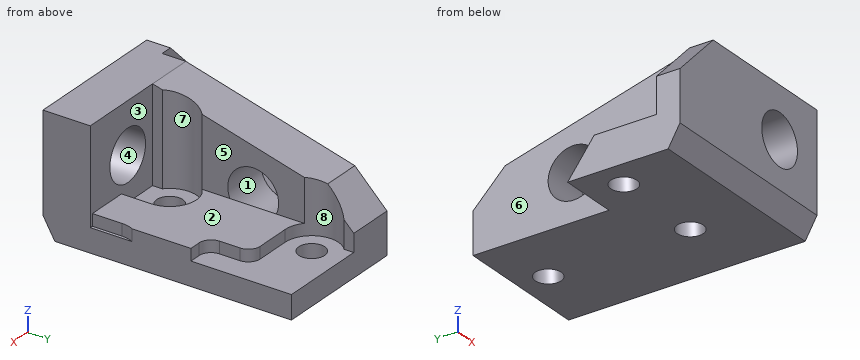
```python
from build123d import *

# Parameters (mm, degrees)
SKETCH_1_W               = 23
SKETCH_1_H               = 17
SKETCH_1_R               = 1.1
EXTRUDE_1_DEPTH          = 3
EXTRUDE_2_DEPTH          = 6
CUT_EXTRUDE_1_DEPTH      = 23.349496639
CUT_EXTRUDE_1_DEPTH_BACK = 1
SKETCH_3_R               = 2.25
CUT_EXTRUDE_2_REACH      = 24.349
SKETCH_4_W               = 4.5
SKETCH_4_H               = 17
CUT_EXTRUDE_3_DEPTH      = 2
SKETCH_6_R               = 2.15
CUT_EXTRUDE_4_DEPTH      = 4
SKETCH_7_W               = 16.5
SKETCH_7_H               = 10
EXTRUDE_3_DEPTH          = 4
SKETCH_8_R               = 2.15
CUT_EXTRUDE_5_DEPTH      = 4
CHAMFER_1_SIZE           = 1
CHAMFER_1_SIZE2          = 1.732050808
CHAMFER_2_SIZE           = 4
CUT_EXTRUDE_6_DEPTH      = 1
FILLET_1_R               = 2
CUT_EXTRUDE_7_REACH      = 21.881
FILLET_2_R               = 1
CHAMFER_3_SIZE           = 2
CHAMFER_3_SIZE2          = 2.813680863
CUT_EXTRUDE_8_REACH      = 27.729
SKETCH_11_W              = 5
SKETCH_11_H              = 10
EXTRUDE_4_DEPTH          = 5
CUT_EXTRUDE_9_REACH      = 21.222
SKETCH_13_R              = 1.1
SKETCH_14_R              = 2.25
CUT_EXTRUDE_10_DEPTH     = 1
EXTRUDE_6_REACH          = 26.135
FILLET_3_R               = 2
SKETCH_15_W              = 5
SKETCH_15_H              = 2
EXTRUDE_5_DEPTH          = 7
CUT_EXTRUDE_11_DEPTH     = 5
CHAMFER_4_SIZE           = 4


with BuildPart() as part:
    # 草图1 → 凸台-拉伸1 (new body)
    with BuildSketch(Plane.XY):
        with Locations((4, 6)):
            Rectangle(SKETCH_1_W, SKETCH_1_H)
        Circle(SKETCH_1_R, mode=Mode.SUBTRACT)
        with Locations((8, 0)):
            Circle(SKETCH_1_R, mode=Mode.SUBTRACT)
        with Locations((0, 12)):
            Circle(SKETCH_1_R, mode=Mode.SUBTRACT)
        with Locations((8, 12)):
            Circle(SKETCH_1_R, mode=Mode.SUBTRACT)
    extrude(amount=EXTRUDE_1_DEPTH)

    # 草图2 → 凸台-拉伸2 (add)
    with BuildSketch(Plane.ZY.offset(7.5)):
        Polygon((5.5, 14.5), (10, -2.5), (5.5, -2.5), (0, -2.5), (0, 14.5), align=None)
    extrude(amount=-EXTRUDE_2_DEPTH)

    # 草图3 → 切除-拉伸1 (cut, two sides: drawn at the far end of the back side and taken through both)
    with BuildSketch(Plane.XY.offset(3).offset(-CUT_EXTRUDE_1_DEPTH_BACK)):
        with Locations(Location((0, 12, 0), (0, 0, 228.189685104))):
            Circle(SKETCH_3_R)
        with Locations((8, 12)):
            Circle(SKETCH_3_R)
        with Locations(Location((0, 0, 0), (0, 0, 131.810314896))):
            Circle(SKETCH_3_R)
        with Locations((8, 0)):
            Circle(SKETCH_3_R)
    extrude(amount=CUT_EXTRUDE_1_DEPTH + CUT_EXTRUDE_1_DEPTH_BACK, mode=Mode.SUBTRACT)

    # 草图4 → 切除-拉伸2 (cut, up to next)
    with BuildSketch(Plane.XY.offset(3), mode=Mode.PRIVATE) as cut_extrude_2_sk1:
        with Locations((13.25, 6)):
            Rectangle(SKETCH_4_W, SKETCH_4_H)
    cut_extrude_2_tool1 = extrude(cut_extrude_2_sk1.sketch, amount=-CUT_EXTRUDE_2_REACH, mode=Mode.PRIVATE) & part.part
    add(cut_extrude_2_tool1.solids().sort_by_distance((13.25, 6, 3))[0], mode=Mode.SUBTRACT)

    # 草图5 → 切除-拉伸3 (cut)
    with BuildSketch(Plane.ZY.offset(7.5)):
        Polygon((0, 14.5), (0, -2.5), (10, -2.5), (5.5, 14.5), align=None)
    extrude(amount=-CUT_EXTRUDE_3_DEPTH, mode=Mode.SUBTRACT)

    # 草图6 → 切除-拉伸4 (cut)
    with BuildSketch(Plane.ZY.offset(5.5)):
        with Locations(Location((3.875, 6, 0), (0, 0, 270))):
            Circle(SKETCH_6_R)
    extrude(amount=-CUT_EXTRUDE_4_DEPTH, mode=Mode.SUBTRACT)

    # 草图7 → 凸台-拉伸3 (add)
    with BuildSketch(Plane.XZ.offset(2.5)):
        with Locations((2.75, 5)):
            Rectangle(SKETCH_7_W, SKETCH_7_H)
    extrude(amount=EXTRUDE_3_DEPTH)

    # 草图8 → 切除-拉伸5 (cut)
    with BuildSketch(Plane.XZ.offset(6.5)):
        with Locations(Location((1.5, 5.7, 0), (0, 0, 270))):
            Circle(SKETCH_8_R)
    extrude(amount=-CUT_EXTRUDE_5_DEPTH, mode=Mode.SUBTRACT)

    # 倒角1
    chamfer_1_edges = [part.edges().sort_by_distance(p)[0] for p in [
        (2.75, -6.5, 0),
    ]]
    chamfer_1_side = [part.faces().sort_by_distance(p)[0] for p in [
        (2.692629218, 3.908206749, 0),
    ]]
    chamfer(chamfer_1_edges, length=CHAMFER_1_SIZE, length2=CHAMFER_1_SIZE2, reference=chamfer_1_side[0])

    # 倒角2
    chamfer_2_edges = [part.edges().sort_by_distance(p)[0] for p in [
        (11, -4.5, 10),
    ]]
    chamfer(chamfer_2_edges, length=CHAMFER_2_SIZE)

    # 草图9 → 切除-拉伸6 (cut)
    with BuildSketch(Plane.XY.offset(3)):
        with BuildLine():
            Line((-1.5, 13.677050983), (-1.5, 14.5))
            Line((-1.5, 14.5), (2.25, 14.5))
            Line((2.25, 14.5), (2.25, 12))
            ThreePointArc((2.25, 12), (0.918558654, 14.053959591), (-1.5, 13.677050983))
        make_face()
        with BuildLine():
            Line((5.75, 12), (5.75, 14.5))
            Line((5.75, 14.5), (11, 14.5))
            Line((11, 14.5), (11, 9.75))
            Line((11, 9.75), (8, 9.75))
            ThreePointArc((8, 9.75), (9.590990258, 13.590990258), (5.75, 12))
        make_face()
        with BuildLine():
            Line((2.25, 0), (2.25, -2.5))
            Line((2.25, -2.5), (-1.5, -2.5))
            Line((-1.5, -2.5), (-1.5, -1.677050983))
            ThreePointArc((-1.5, -1.677050983), (0.918558654, -2.053959591), (2.25, 0))
        make_face()
        with BuildLine():
            Line((5.75, 0), (5.75, -2.5))
            Line((5.75, -2.5), (11, -2.5))
            Line((11, -2.5), (11, 2.25))
            Line((11, 2.25), (8, 2.25))
            ThreePointArc((8, 2.25), (9.590990258, -1.590990258), (5.75, 0))
        make_face()
    extrude(amount=-CUT_EXTRUDE_6_DEPTH, mode=Mode.SUBTRACT)

    # 圆角1
    fillet_1_edges = [part.edges().sort_by_distance(p)[0] for p in [
        (11, 14.5, 1),
    ]]
    fillet(fillet_1_edges, radius=FILLET_1_R)

    # 草图10 → 切除-拉伸7 (cut, up to next)
    with BuildSketch(Plane.XY.offset(2), mode=Mode.PRIVATE) as cut_extrude_7_sk1:
        with BuildLine():
            Line((4, 14.5), (11, 14.5))
            Line((11, 14.5), (11, 6))
            Line((11, 6), (4, 6))
            Line((4, 6), (4, 9.75))
            Line((4, 9.75), (0, 9.75))
            ThreePointArc((0, 9.75), (1.590990258, 10.409009742), (2.25, 12))
            Line((2.25, 12), (2.25, 14.5))
            Line((2.25, 14.5), (4, 14.5))
        make_face()
    cut_extrude_7_tool1 = extrude(cut_extrude_7_sk1.sketch, amount=CUT_EXTRUDE_7_REACH, mode=Mode.PRIVATE) & part.part
    add(cut_extrude_7_tool1.solids().sort_by_distance((6.881457, 10.476255, 2))[0], mode=Mode.SUBTRACT)

    # 圆角2
    fillet_2_edges = [part.edges().sort_by_distance(p)[0] for p in [
        (4, 9.75, 2.5),
        (4, 6, 2.5),
    ]]
    fillet(fillet_2_edges, radius=FILLET_2_R)

    # 倒角3
    chamfer_3_edges = [part.edges().sort_by_distance(p)[0] for p in [
        (-3.5, 14.5, 5.5),
    ]]
    chamfer_3_side = [part.faces().sort_by_distance(p)[0] for p in [
        (0.040697674, 14.5, 1.895348837),
    ]]
    chamfer(chamfer_3_edges, length=CHAMFER_3_SIZE, length2=CHAMFER_3_SIZE2, reference=chamfer_3_side[0])

    # 草图11 → 切除-拉伸8 (cut, up to next)
    with BuildSketch(Plane.XZ.offset(6.5), mode=Mode.PRIVATE) as cut_extrude_8_sk1:
        with Locations((8.5, 5)):
            Rectangle(SKETCH_11_W, SKETCH_11_H)
    cut_extrude_8_tool1 = extrude(cut_extrude_8_sk1.sketch, amount=-CUT_EXTRUDE_8_REACH, mode=Mode.PRIVATE) & part.part
    add(cut_extrude_8_tool1.solids().sort_by_distance((8.5, -6.5, 5))[0], mode=Mode.SUBTRACT)

    # 草图12 → 凸台-拉伸4 (add)
    with BuildSketch(Plane.ZY.offset(5.5)):
        Polygon((0, -5.5), (1.732050808, -6.5), (3, -6.5), (3, 1.5), (0, 1.5), align=None)
    extrude(amount=EXTRUDE_4_DEPTH)

    # 草图13 → 切除-拉伸9 (cut, up to next)
    with BuildSketch(Plane.XY.offset(3), mode=Mode.PRIVATE) as cut_extrude_9_sk1:
        with Locations((-8, 0)):
            Circle(SKETCH_13_R)
    cut_extrude_9_tool1 = extrude(cut_extrude_9_sk1.sketch, amount=-CUT_EXTRUDE_9_REACH, mode=Mode.PRIVATE) & part.part
    add(cut_extrude_9_tool1.solids().sort_by_distance((-8, 0, 3))[0], mode=Mode.SUBTRACT)

    # 草图14 → 切除-拉伸10 (cut)
    with BuildSketch(Plane.XY.offset(3)):
        with Locations((-8, 0)):
            Circle(SKETCH_14_R)
    extrude(amount=-CUT_EXTRUDE_10_DEPTH, mode=Mode.SUBTRACT)

    # 凸台-拉伸6: up to this face of the body (flat: up to its plane)
    extrude_6_end = Plane(part.part.faces().sort_by_distance((-5.5, 3.356262463, 4.741493194))[0])
    # 草图16 → 凸台-拉伸6 (add, up to the picked face)
    with BuildSketch(Plane.ZY.offset(10.5), mode=Mode.PRIVATE) as extrude_6_sk1:
        Polygon((2, 1.5), (0, 3), (0, 1.5), align=None)
    extrude_6_tool1 = split(extrude(extrude_6_sk1.sketch, amount=-EXTRUDE_6_REACH, mode=Mode.PRIVATE), bisect_by=extrude_6_end, keep=Keep.BOTH, mode=Mode.PRIVATE)
    add(extrude_6_tool1.solids().sort_by(Axis((-10.5, 2, 0.666667), (1, 0, 0)))[0])

    # 圆角3
    # the kernel refuses this fillet: 2 mm, written as the material it takes off along each edge
    with BuildSketch(Plane(origin=(-10.5, 1.5, 7.042393307), x_dir=(1, 0, 0), z_dir=(0, 0, -1))) as fillet_3_piece_1_section:
        with BuildLine():
            CenterArc((2, 1.616957323), FILLET_3_R, 180, 53.947557716)
            Line((0, 1.616957323), (0, 0))
            Line((0, 0), (0.822949017, 0))
        make_face()
    fillet_3_piece_1 = extrude(amount=9.084786613, mode=Mode.PRIVATE)
    fillet_3_piece_1 = split(fillet_3_piece_1, bisect_by=Plane(origin=(-10.039236146, 1.139870627, 2.480172498), z_dir=(0, 0.8000000000000002, 0.6)), keep=Keep.TOP, mode=Mode.PRIVATE)
    add(fillet_3_piece_1, mode=Mode.SUBTRACT)

    # 草图15 → 凸台-拉伸5 (add)
    with BuildSketch(Plane.XY.offset(3)):
        with Locations((-8, -5.5)):
            Rectangle(SKETCH_15_W, SKETCH_15_H)
    extrude(amount=EXTRUDE_5_DEPTH)

    # 草图17 → 切除-拉伸11 (cut)
    with BuildSketch(Plane.ZY.offset(10.5)):
        Polygon((2, 1.5), (3, 0.75), (3, 1.5), align=None)
    extrude(amount=-CUT_EXTRUDE_11_DEPTH, mode=Mode.SUBTRACT)

    # 倒角4
    chamfer_4_edges = [part.edges().sort_by_distance(p)[0] for p in [
        (-10.5, -5.5, 10),
    ]]
    chamfer(chamfer_4_edges, length=CHAMFER_4_SIZE)


solid = part.part
```
Work out the finished part from the listing and answer in its coordinate system (mm). Face numbers are marked on the shaded views. A direction names the side the tool comes from. Coordinates: 2 decimals unless noted, no trailing zeros. Write each loop counter-clockwise with the first axis right and the second up, starting at its lowest first coordinate (ties: lowest second). Pieces come first, ordered by that corner, then holes. Notation, with made-up numbers: (-9.75, -13.75) - (38.25, -13.75) arc R26 cw to (38.25, 2.25) - close; hole circle Ø1 at (-27.5, 22). An arc over 180 degrees is marked (long way). Answer as a JSON object with one key per item and string values.
Q1. Given pin 1 Ø1.5 at (x, z) = (-9, 7) entering from +Y; pin 2 Ø3 at (y, z) = (0, 7) entering from +X; pin 3 Ø8.5 at (x, y) = (4, 2.5) entering from +Z, each flat-ended and moving along its own axis, determine where each tip first touches the part or whether it passes through.
Results list:
{"pin 1": "stops at y = -4.5", "pin 2": "stops at x = -1.68", "pin 3": "stops at z = 3"}
Q2. Consider L1, parallel to X at y = 12, z = 1.35; L2, parallel to Z at x = 5, y = 1.25; L3, parallel to Y at x = 5.25, z = 9.75. Determine where each line is inside the solid, lowest interval first. Write a range as from..to.
Results list:
{"L1": "x = -5.5..-1.1, 1.1..6", "L2": "z = 0..3", "L3": "y = -6.5..-2.5"}
Q3. Find section D-D (z = 5.5). Write down the section's boundary in (x, y), plus the area to 3 significant figures.
Results list:
{"outline": "(-10.5, -6.5) - (-0.64, -6.5) - (-0.64, -2.5) - (-1.5, -2.5) - (-1.5, -1.68) arc R2.25 cw to (-1.5, 1.68) - (-1.5, 4.59) - (-5.5, 4.59) - (-5.5, -4.5) - (-10.5, -4.5) - close; (-5.5, 7.41) - (-1.5, 7.41) - (-1.5, 10.32) arc R2.25 cw to (-2.19, 12.5) - (-5.5, 12.5) - close; (3.64, -6.5) - (6, -6.5) - (6, -2.5) - (3.64, -2.5) - close", "area": "84.6 mm^2"}
Q4. Find section A-A (x = 1.5). Write down the section's boundary in (y, z), plus the area to 3 significant figures.
Results list:
{"outline": "(-6.5, 1.73) - (-5.5, 0) - (14.5, 0) - (14.5, 2) - (9.75, 2) - (9.75, 3) - (1.68, 3) - (1.68, 2) - (-2.5, 2) - (-2.5, 3.55) - (-6.5, 3.55) - close; (-6.5, 7.85) - (-2.5, 7.85) - (-2.5, 10) - (-6.5, 10) - close", "area": "64.0 mm^2"}
Q5. Which of the six approach directions +Z, -Z, +X, -X, +Y, -Y give full straight-line access (tool end or side, diameter ignored) to the marked faces 5, 6, 7 and 8?
Results list:
{"face 5": "+Z, +X, +Y", "face 6": "+Z, -X, +Y", "face 7": "+Z", "face 8": "+Z, +X"}
Q6. Find section B-B (z = 3.25). Write down the section's boundary in (x, y), plus the area to 3 significant figures.
Results list:
{"outline": "(-10.5, -6.5) - (6, -6.5) - (6, -2.5) - (-1.5, -2.5) - (-1.5, -1.68) arc R2.25 cw to (-1.5, 1.68) - (-1.5, 3.94) - (-5.5, 3.94) - (-5.5, -4.5) - (-10.5, -4.5) - close; (-5.5, 8.06) - (-1.5, 8.06) - (-1.5, 10.32) arc R2.25 cw to (-1.5, 13.68) - (-1.5, 14.5) - (-5.5, 14.5) - close", "area": "104 mm^2"}
Q7. Find section C-C (y = -0.5). Write down the section's boundary in (x, z), plus the area to 3 significant figures.
Results list:
{"outline": "(-10.5, 0) - (-8.98, 0) - (-8.98, 2) - (-10.19, 2) - (-10.19, 3) - (-10.5, 3) - close; (-7.02, 0) - (-0.98, 0) - (-0.98, 2) - (-2.19, 2) - (-2.19, 9.47) - (-5.5, 9.47) - (-5.5, 3) - (-5.81, 3) - (-5.81, 2) - (-7.02, 2) - close; (0.98, 0) - (6, 0) - (6, 2) - (5.75, 2) - (5.75, 3) - (2.25, 3) - (2.25, 2) - (0.98, 2) - close", "area": "54.0 mm^2"}
Q8. For a pull along Z with two mould halves and no side action, classify the marked faces 1, 2, 3 and 4 as pulls with the +Z half, pulls with the -Z half, needs draft (parallel to the pull), parting line crosses it, or undercut.
Results list:
{"face 1": "undercut", "face 2": "pulls with the +Z half", "face 3": "needs draft", "face 4": "undercut"}
